For this review, use the dimensioned drawing (mm, ordinates from the lowest corner) and the shaded views. Coordinates: 2 decimals unless noted, no trailing zeros. Write each loop counter-clockwise with the first axis right and the second up, starting at its lowest first coordinate (ties: lowest second). Pieces come first, ordered by that corner, then holes. Notation, with made-up numbers: (32, -24.5) - (61, -24.5) arc R22 cw to (61, 5.5) - close; hole circle Ø9 at (-18.5, -14). An arc over 180 degrees is marked (long way). Use one line per item in the form item = value. Start each with the question number.
1) For L1, parallel to Y at x = 35, z = 0.2; L2, parallel to Y at x = 24, z = 0.1 (1 decimal); L3, parallel to X at y = 23, z = 0.8, list the stretches that pass through material, from the lowest coordinate up. Write a range as from..to.
2) We need section B-B (z = 0.25). Count the separate pieces of the cut face and the enclosed holes in it, plus the area to 3 significant figures.
3) We need section D-D (y = 8.5). Give the boundary of the cut face in (x, z).
4) We need section A-A (x = 35). Give the boundary of the cut face in (y, z).
5) We need section C-C (y = 22.5). Give the boundary of the cut face in (x, z).
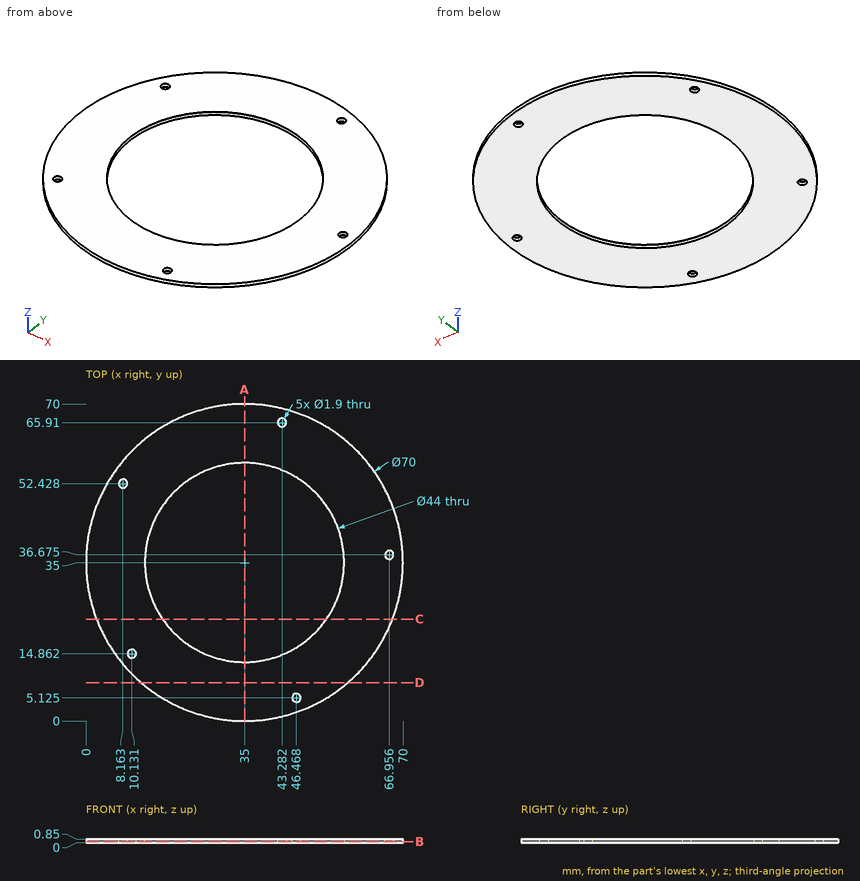
Determined:
q1.L1 = 0..13, 57..70
q1.L2 = 1.8..15.9, 54.1..68.2
q1.L3 = 2.12..16.56, 53.44..67.88
q2.separate_pieces = 1
q2.enclosed_holes = 6
q2.area = 2,310 mm²
q3.outline = (12.14, 0) - (57.86, 0) - (57.86, 0.85) - (12.14, 0.85) - close
q4.outline = (0, 0) - (13, 0) - (13, 0.85) - (0, 0.85) - close; (57, 0) - (70, 0) - (70, 0.85) - (57, 0.85) - close
q5.outline = (2.31, 0) - (16.9, 0) - (16.9, 0.85) - (2.31, 0.85) - close; (53.1, 0) - (67.69, 0) - (67.69, 0.85) - (53.1, 0.85) - close
